from build123d import *

# Parameters (mm, degrees)
RESSALTO_EXTRUS_O1_DEPTH = 160
ESBO_O2_W                = 7.6
ESBO_O2_H                = 120
CORTE_EXTRUS_O1_DEPTH    = 30
CORTE_EXTRUS_O2_DEPTH    = 30
F_3DSKETCH3_R            = 2
CORTE_EXTRUS_O3_DEPTH    = 70


with BuildPart() as part:
    # Esboço1 → Ressalto-extrusão1 (new body)
    with BuildSketch(Plane.XY):
        with BuildLine():
            Line((-3.8, 21.821375341), (-3.8, -98.178624659))
            Line((-3.8, -98.178624659), (-5.7, -98.178624659))
            Line((-5.7, -98.178624659), (-5.360626179, -99.63308389))
            ThreePointArc((-5.360626179, -99.63308389), (-4.656141559, -100.745296045), (-3.41294376, -101.178624659))
            Line((-3.41294376, -101.178624659), (3.41294376, -101.178624659))
            ThreePointArc((3.41294376, -101.178624659), (4.656141559, -100.745296045), (5.360626179, -99.63308389))
            Line((5.360626179, -99.63308389), (5.7, -98.178624659))
            Line((5.7, -98.178624659), (3.8, -98.178624659))
            Line((3.8, -98.178624659), (3.8, 21.821375341))
            Line((3.8, 21.821375341), (5.7, 21.821375341))
            Line((5.7, 21.821375341), (4.013268169, 24.033911877))
            ThreePointArc((4.013268169, 24.033911877), (3.310139149, 24.613730366), (2.422747768, 24.821375341))
            Line((2.422747768, 24.821375341), (-2.297792791, 24.821375341))
            ThreePointArc((-2.297792791, 24.821375341), (-3.27177376, 24.568189891), (-3.999156919, 23.872736414))
            Line((-3.999156919, 23.872736414), (-5.266799243, 21.821375341))
            Line((-5.266799243, 21.821375341), (-3.8, 21.821375341))
        make_face()
    extrude(amount=RESSALTO_EXTRUS_O1_DEPTH)

    # Esboço2 → Corte-extrusão1 (cut)
    with BuildSketch(Plane.XY):
        with Locations((0, -38.178624659)):
            Rectangle(ESBO_O2_W, ESBO_O2_H)
    extrude(amount=CORTE_EXTRUS_O1_DEPTH, mode=Mode.SUBTRACT)

    # 3DSketch2 → Corte-extrusão2 (cut)
    with BuildSketch(Plane(origin=(-3.8, 21.821375341, 160), x_dir=(0.0632066956560733, -0.9980004577274705, 0), z_dir=(0, 0, -1))):
        Polygon((0, 0), (0.480370887, -7.584803479), (120.240425814, 0), (119.760054927, 7.584803479), align=None)
    extrude(amount=CORTE_EXTRUS_O2_DEPTH, mode=Mode.SUBTRACT)

    # 3DSketch3 → Corte-extrusão3 (cut)
    with BuildSketch(Plane(origin=(3.8, -38.178624659, 80), x_dir=(0, 0.7676852805184269, 0.6408270516101394), z_dir=(1, 0, 0))):
        with Locations(Location((0, 0, 0), (0, 0, 140.146481665))):
            Circle(F_3DSKETCH3_R)
        with Locations(Location((23.030558416, -19.224811548, 0), (0, 0, 140.146481665))):
            Circle(F_3DSKETCH3_R)
        with Locations(Location((-23.030558416, 19.224811548, 0), (0, 0, 140.146481665))):
            Circle(F_3DSKETCH3_R)
        with Locations(Location((-39.051234706, 0.032679535, 0), (0, 0, 140.146481665))):
            Circle(F_3DSKETCH3_R)
        with Locations(Location((-16.02067629, -19.192132013, 0), (0, 0, 140.146481665))):
            Circle(F_3DSKETCH3_R)
        with Locations(Location((7.009882125, -38.416943561, 0), (0, 0, 140.146481665))):
            Circle(F_3DSKETCH3_R)
        with Locations(Location((-6.982602808, 38.449623097, 0), (0, 0, 140.146481665))):
            Circle(F_3DSKETCH3_R)
        with Locations(Location((16.047955607, 19.224811548, 0), (0, 0, 140.146481665))):
            Circle(F_3DSKETCH3_R)
        with Locations(Location((39.078514023, 0, 0), (0, 0, 140.146481665))):
            Circle(F_3DSKETCH3_R)
    extrude(amount=-CORTE_EXTRUS_O3_DEPTH, mode=Mode.SUBTRACT)


solid = part.part
Can you work these out from the model? Positions are in its coordinate system, mm. A direction names the side the tool comes from. Give positions to 0.01 mm unless a question says otherwise; leave off trailing zeros. Loops run counter-clockwise (first coordinate to the right, second up) from the corner with the lowest first, then second, coordinate; pieces in that order, holes last. Notation, with made-up numbers: M 13.5,57.5 L 42.5,57.5 A28 ccw 42.5,92.5 Z; hole C 1,41.25 d6. An arc over 180 degrees is marked long. One line per item, written item: value. Start each with the question number.
1) If we section it at A-A, the plane z = 55: Write out the boundary of the cut face in (x, y).
2) If we section it at B-B, the plane x = 0: Give the number of separate pieces and of enclosed holes in the cut face, and give its area (3 significant figures).
3) On a 3-axis mill with a long thin cutter (end or side, diameter ignored), from which of +Z, -Z, +X, -X, +Y, -Y can I reach the whole of each face in a straight line? I mean faces 1 (the face through (-3.8, -37, 68)), 2 (the face through (3.8, -39, 68)), 3 (the face through (0, -37, 130)), 4 (the face through (0, -37, 30)). Say none if no direction works.
4) Thinking about a two-plate mould opening in Y: for faces 5 (the face through (0.053, -37.918, 78.017)), 6 (the face through (0, -101.179, 79)), 7 (the face through (0, 24.821, 79)), which applies, +Y half, -Y half, draft (parallel to the pull), parting line (faces both ways), or undercut?
5) If we section it at C-C, the plane z = 96: Write out the boundary of the cut face in (x, y), and give its area (3 significant figures).
6) If I drill on line 1 (Y direction, x = 2.5, z = 104.5); line 2 (Z direction, x = -1.25, y = -67); line 3 (Y direction, x = -1.25, z = 153), over which ranges is the centre line in solid material (lowest first)? Write a range as [from, to].
7) If we section it at D-D, the plane y = -48.5: Write out the boundary of the cut face in (x, z).
8) I'm going to push flat-ended pins straight in: pin 1 (5 mm diameter, centred on y = -44.5, z = 115, fed in from +X); pin 2 (4 mm diameter, centred on x = 1, y = -23.5, fed in from +Z); pin 3 (5 mm diameter, centred on y = -68.18, z = 80, fed in from -X). Where does each tip first touch, or does it pass through?
Completed:
1. outline: M -5.7,-98.18 L -5.36,-99.63 A2 ccw -3.41,-101.18 L 3.41,-101.18 A2 ccw 5.36,-99.63 L 5.7,-98.18 L 3.8,-98.18 L 3.8,-70.18 L -3.8,-70.18 L -3.8,-98.18 Z; M -5.27,21.82 L -3.8,21.82 L -3.8,-6.18 L 3.8,-6.18 L 3.8,21.82 L 5.7,21.82 L 4.01,24.03 A2 ccw 2.42,24.82 L -2.3,24.82 A2 ccw -4,23.87 Z; M -3.8,-66.18 L 3.8,-66.18 L 3.8,-40.18 L -3.8,-40.18 Z; M -3.8,-36.18 L 3.8,-36.18 L 3.8,-10.18 L -3.8,-10.18 Z
2. separate pieces: 1
2. enclosed holes: 9
2. area: 12,800 mm^2
3. face 1: +Z, -Z, -X
3. face 2: +Z, -Z, +X
3. face 3: +Z, +X, -X
3. face 4: -Z, +X, -X
4. face 5: undercut
4. face 6: -Y half
4. face 7: +Y half
5. outline: M -5.7,-98.18 L -5.36,-99.63 A2 ccw -3.41,-101.18 L 3.41,-101.18 A2 ccw 5.36,-99.63 L 5.7,-98.18 L 3.8,-98.18 L 3.8,21.82 L 5.7,21.82 L 4.01,24.03 A2 ccw 2.42,24.82 L -2.3,24.82 A2 ccw -4,23.87 L -5.27,21.82 L -3.8,21.82 L -3.8,-98.18 Z
5. area: 969 mm^2
6. line 1: y = [-101.18, -70.1], [-66.25, -40.1], [-36.25, -10.1], [-6.25, 24.82]
6. line 2: z = [30, 53.38], [56.62, 78.38], [81.62, 103.43], [106.66, 130]
6. line 3: y = [-101.18, -98.18], [21.82, 24.82]
7. outline: M -3.8,30 L 3.8,30 L 3.8,130 L -3.8,130 Z
8. pin 1: stops at x = 3.8
8. pin 2: stops at z = 130
8. pin 3: stops at x = -3.8
